Geometry check sheet. Reference: drawing and pictorial views, mm from the part's lowest x, y, z. A direction names the side the tool comes from. Give positions to 0.01 mm unless a question says otherwise; leave off trailing zeros. Loops run counter-clockwise (first coordinate to the right, second up) from the corner with the lowest first, then second, coordinate; pieces in that order, holes last. Notation, with made-up numbers: (24.25, 89.25) -> (79.25, 89.25) arc R23 ccw to (79.25, 112.25) -> close; hole circle Ø5 at (78, 11). An arc over 180 degrees is marked (long way). Answer in a Markdown table with one row per item. Add a question column.
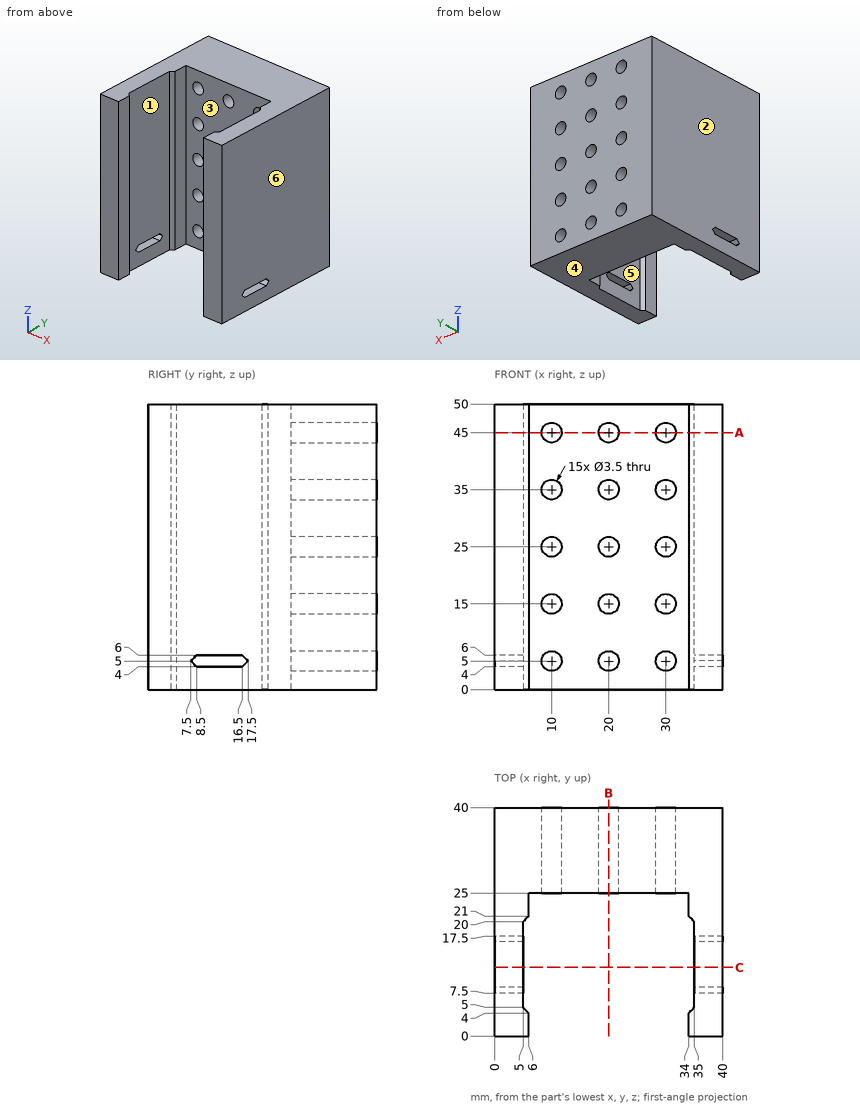
1. Release check for a two-part mould opening along X. For the marked faces 4, 5 and 6 record: released by +X, released by -X, zero draft, split by the parting line, or undercut.
2. Access from +Z, -Z, +X, -X, +Y, -Y to the whole of each face (thin tool, end or side, straight path). Record for the marked faces 1, 2 and 3.
3. Sectioned sample at C-C (y = 12). Enter the section's corners in (x, z).
4. Gauge pin test, flat end, axial feed: pin 1 Ø5.5 at (x, z) = (30, 15) entering from -Y. Record the tip position at first contact, or that the pin passes through.
5. Sectioned sample at B-B (x = 20). Enter the section's corners in (y, z).
6. Material ranges on L1, parallel to X at y = 35.5, z = 45; L2, parallel to X at y = 23, z = 15; L3, parallel to X at y = 16.5, z = 27, recorded low to high. Write a range as from..to.
7. Sectioned sample at A-A (z = 45). Count the separate pieces of the cut face and the enclosed holes in it.
Response:
| question | item | result |
|---|---|---|
| 1 | face 4 | zero draft |
| 1 | face 5 | undercut |
| 1 | face 6 | released by +X |
| 2 | face 1 | +Z, -Z |
| 2 | face 2 | +Z, -Z, -X, +Y, -Y |
| 2 | face 3 | +Z, -Z, -Y |
| 3 | outline | (0, 0) -> (5, 0) -> (5, 4) -> (0, 4) -> close; (0, 6) -> (5, 6) -> (5, 50) -> (0, 50) -> close; (35, 0) -> (40, 0) -> (40, 4) -> (35, 4) -> close; (35, 6) -> (40, 6) -> (40, 50) -> (35, 50) -> close |
| 4 | pin 1 | stops at y = 25 |
| 5 | outline | (25, 0) -> (40, 0) -> (40, 3.25) -> (25, 3.25) -> close; (25, 6.75) -> (40, 6.75) -> (40, 13.25) -> (25, 13.25) -> close; (25, 16.75) -> (40, 16.75) -> (40, 23.25) -> (25, 23.25) -> close; (25, 26.75) -> (40, 26.75) -> (40, 33.25) -> (25, 33.25) -> close; (25, 36.75) -> (40, 36.75) -> (40, 43.25) -> (25, 43.25) -> close; (25, 46.75) -> (40, 46.75) -> (40, 50) -> (25, 50) -> close |
| 6 | L1 | x = 0..8.25, 11.75..18.25, 21.75..28.25, 31.75..40 |
| 6 | L2 | x = 0..6, 34..40 |
| 6 | L3 | x = 0..5, 35..40 |
| 7 | separate pieces | 4 |
| 7 | enclosed holes | 0 |
